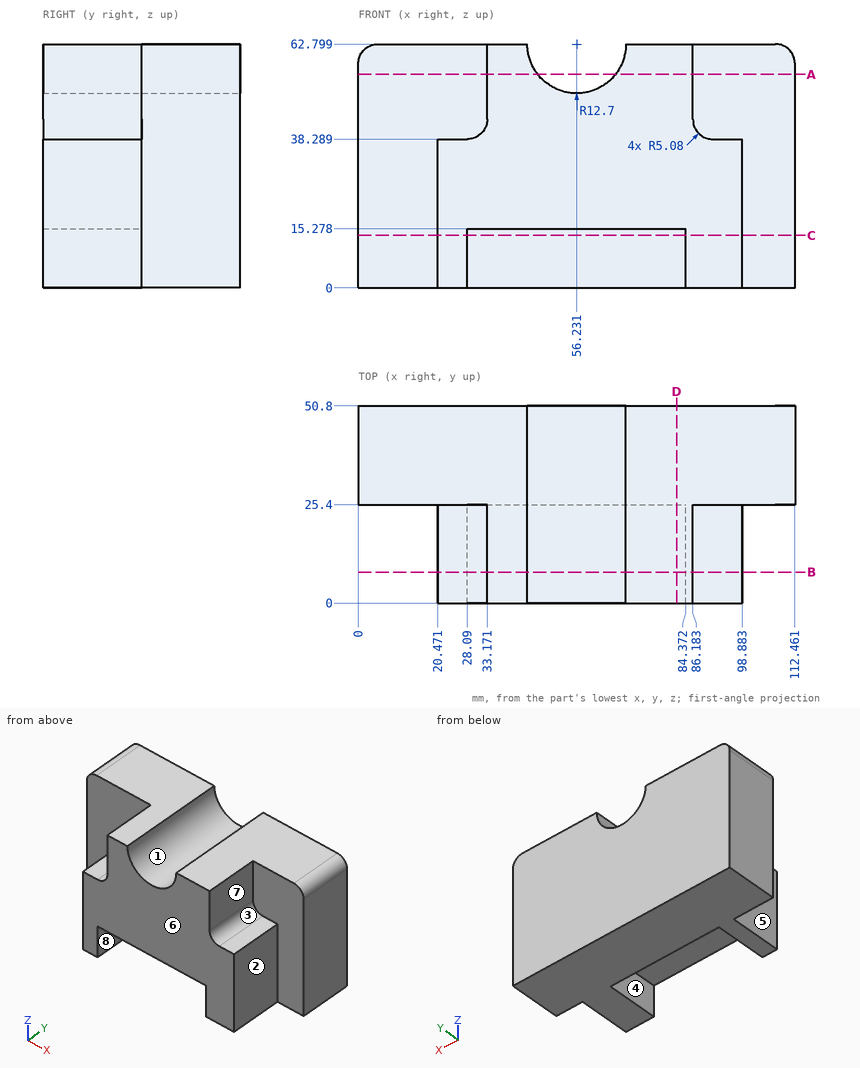
Could you check a few things on this drawing? It's one solid part, dimensions in mm from its lowest x, y, z. A direction names the side the tool comes from. Give positions to 0.01 mm unless a question says otherwise; leave off trailing zeros. Order: outer loops, then holes, each group sorted by start corner. A loop starts at its lowest first (then second) coordinate and runs counter-clockwise, first axis right, second up. Notation, with made-up numbers: M 26.25,-24 L 77.25,-24 A20 ccw 77.25,-18 Z; hole C 53,-29 d3. An arc over 180 degrees is marked long. Use one line per item in the form item = value. Start each with the question number.
Item 1: Will these pins go through, and if not, where does the flat tip stop? pin 1 Ø12.5 at (y, z) = (18.5, 19.5) entering from +X; pin 2 Ø7.5 at (y, z) = (18.5, 14) entering from -X; pin 3 Ø12.5 at (x, y) = (49, 16) entering from -Z.
Item 2: We'd pull the mould along X, two halves only. Please class the marked faces 6, 7 and 8: +X half, -X half, draft (parallel to the pull), parting line (faces both ways), or undercut.
Item 3: If we section it at B-B (y = 8): Write out the boundary of the cut face in (x, z), then the cut area to 3 significant figures.
Item 4: If we section it at A-A (z = 55): Write out the boundary of the cut face in (x, y).
Item 5: If I drill on line 1 along X through (y, z) = (15, 6); line 2 along Z through (x, y) = (42, 9.5); line 3 along X through (y, z) = (7, 53.5) (1 decimal), over which ranges is the centre line in solid material (lowest first)?
Item 6: If we section it at D-D (x = 82): Write out the boundary of the cut face in (y, z).
Item 7: If we section it at C-C (z = 13.5): Write out the boundary of the cut face in (x, y).
Item 8: For the marked faces 1, 2, 3, 4 and 5, which set-ups out of +Z, -Z, +X, -X, +Y, -Y let a thin tool reach every point of the face, with its end or its side?
Outcome:
q1.pin_1 = 98.88
q1.pin_2 = 20.47
q1.pin_3 = 15.28
q2.face_6 = draft
q2.face_7 = +X half
q2.face_8 = undercut
q3.outline = M 20.47,0 L 28.09,0 L 28.09,15.28 L 84.37,15.28 L 84.37,0 L 98.88,0 L 98.88,38.29 L 91.26,38.29 A5.08 cw 86.18,43.37 L 86.18,62.8 L 68.93,62.8 A12.7 cw 43.53,62.8 L 33.17,62.8 L 33.17,43.37 A5.08 cw 28.09,38.29 L 20.47,38.29 Z
q3.area = 3,200 mm2
q4.outline = M 0,25.4 L 33.17,25.4 L 33.17,0 L 46.21,0 L 46.21,50.8 L 0,50.8 Z; M 66.25,0 L 86.18,0 L 86.18,25.4 L 112.46,25.4 L 112.46,50.8 L 66.25,50.8 Z
q5.line_1 = 20.47 to 28.09, 84.37 to 98.88
q5.line_2 = 15.28 to 62.8
q5.line_3 = 33.2 to 47.6, 64.9 to 86.2
q6.outline = M 0,15.28 L 25.4,15.28 L 25.4,0 L 50.8,0 L 50.8,62.8 L 0,62.8 Z
q7.outline = M 0,25.4 L 20.47,25.4 L 20.47,0 L 28.09,0 L 28.09,25.4 L 84.37,25.4 L 84.37,0 L 98.88,0 L 98.88,25.4 L 112.46,25.4 L 112.46,50.8 L 0,50.8 Z
q8.face_1 = +Z, +Y, -Y
q8.face_2 = +Z, -Z, +X, -Y
q8.face_3 = +Z, +X, -Y
q8.face_4 = -Z, -Y
q8.face_5 = +Z, -Z, -X, -Y
